Design review of the part built by this model. Coordinates are the model's own, in mm. A direction names the side the tool comes from. Give positions to 0.01 mm unless a question says otherwise; leave off trailing zeros. Loops run counter-clockwise (first coordinate to the right, second up) from the corner with the lowest first, then second, coordinate; pieces in that order, holes last. Notation, with made-up numbers: M -24,5 L 25,5 A21 cw 25,18 Z; hole C 19.25,8.25 d5. An arc over 180 degrees is marked long. Use CSV: the item, a comma, the result in double quotes.
from build123d import *

# Parameters (mm, degrees)
SKETCH1_W           = 295
SKETCH1_H           = 100
SKETCH1_W_2         = 5
SKETCH1_H_2         = 50
BOSS_EXTRUDE1_DEPTH = 5
SKETCH2_W           = 70
SKETCH2_H           = 5
CUT_EXTRUDE1_DEPTH  = 5


with BuildPart() as part:
    # Sketch1 → Boss-Extrude1 (new body)
    with BuildSketch(Plane.XY):
        with Locations((-147.5, 50)):
            Rectangle(SKETCH1_W, SKETCH1_H)
        with Locations((2.5, 50)):
            Rectangle(SKETCH1_W_2, SKETCH1_H_2)
        with Locations((-297.5, 50)):
            Rectangle(SKETCH1_W_2, SKETCH1_H_2)
    extrude(amount=BOSS_EXTRUDE1_DEPTH)

    # Sketch2 → Cut-Extrude1 (cut)
    with BuildSketch(Plane.XY.offset(5)):
        with Locations((-210, 7.5)):
            Rectangle(SKETCH2_W, SKETCH2_H)
        with Locations((-85, 7.5)):
            Rectangle(SKETCH2_W, SKETCH2_H)
    extrude(amount=-CUT_EXTRUDE1_DEPTH, mode=Mode.SUBTRACT)


solid = part.part
(1) We need section B-B on z = 2.75. State the section outline as (x, y) points, then the cut area to 3 significant figures.
A:
outline,"M -300,25 L -295,25 L -295,0 L 0,0 L 0,25 L 5,25 L 5,75 L 0,75 L 0,100 L -295,100 L -295,75 L -300,75 Z; hole M -245,5 L -175,5 L -175,10 L -245,10 Z; hole M -120,5 L -50,5 L -50,10 L -120,10 Z"
area,"29,300 mm²"
(2) Clearance check with flat-ended pins moving along their axes: P1, Ø1.5, axis at y = 91, z = 2, coming from the +X side; P2, Ø2.5, axis at x = 3.5, z = 1.5, coming from the +Y side; P3, Ø2.5, axis at x = 2.5, z = 1.5, coming from the -Y side. State where each tip first meets the part, or that it passes through.
A:
P1,"x = 0"
P2,"y = 75"
P3,"y = 25"
(3) The part is to be moulded in two halves that separate along X. For faces 4 (the flat face through (-295, 12, 2)), 5 (the flat face through (5, 50, 2)), 6 (the flat face through (-245, 7, 3)), say which applies: released by +X, released by -X, zero draft, split by the parting line, or undercut.
A:
face 4,"released by -X"
face 5,"released by +X"
face 6,"undercut"
(4) Wall thickness on line 1 along Y through (x, z) = (-238.5, 4.7); line 2 along X through (y, z) = (88, 1.5): over which ranges is each line inside the solid? List them lowest first. Write a range as [from, to].
A:
line 1,"[0, 5], [10, 100]"
line 2,"[-295, 0]"
(5) We need section C-C on y = 89. State the section outline as (x, z) points.
A:
outline,"M -295,0 L 0,0 L 0,5 L -295,5 Z"
(6) Machinability: for faces 1 (the flat face through (-175, 7, 3)), 2 (the flat face through (-295, 87, 2)), 3 (the flat face through (2, 25, 2)), which of the approach directions +Z, -Z, +X, -X, +Y, -Y give a long, thin tool a straight path to every point of the face, cutting with its end or side? Answer none if there is none.
A:
face 1,"+Z, -Z"
face 2,"+Z, -Z, -X, +Y"
face 3,"+Z, -Z, +X, -Y"
(7) We need section A-A on x = -214. State the section outline as (y, z) points.
A:
outline,"M 0,0 L 5,0 L 5,5 L 0,5 Z; M 10,0 L 100,0 L 100,5 L 10,5 Z"
